The model under review builds one solid part; all positions refer to its coordinate system, in mm. Face numbers are marked on the shaded views. A direction names the side the tool comes from. Coordinates: 2 decimals unless noted, no trailing zeros. Write each loop counter-clockwise with the first axis right and the second up, starting at its lowest first coordinate (ties: lowest second). Pieces come first, ordered by that corner, then holes. Notation, with made-up numbers: (-36.75, 6) - (19.25, 6) arc R27 cw to (19.25, 33) - close; hole circle Ø3 at (-18.5, -5). An arc over 180 degrees is marked (long way). Return JSON: item names as keys, results as strings. Group by question number.
(1) For pin 1 Ø8 at (x, y) = (9, 45) entering from +Z; pin 2 Ø1 at (x, y) = (6.5, 98.5) entering from +Z; pin 3 Ø4 at (x, y) = (3, 37) entering from +Z; pin 4 Ø2.5 at (y, z) = (49.4, 132.79) entering from -X, all flat-tipped, find the tip position at first contact; note any pin that passes through.
(2) We need section C-C on y = 40.5. State the section outline as (x, z) points, then the cut area to 3 significant figures.
(3) Tool access review of the marked faces 4 and 5: name each direction out of +Z, -Z, +X, -X, +Y, -Y from which nothing blocks a thin tool from reaching the whole face with its end or side.
(4) Draft analysis for pull direction Z (two halves, no side actions). For the marked faces 1, 2 and 3, state which applies: released by +Z, released by -Z, zero draft, split by the parting line, or undercut.
(5) We need section A-A on x = 5.25. State the section outline as (y, z) points, then the cut area to 3 significant figures.
(6) To check wall thickness, follow L1, parallel to X at y = 108.5, z = 24; L2, parallel to Z at x = 12.5, y = 75; L3, parallel to Y at x = 1.75, z = 141.5. State the ranges of each line that lie inside material, in increasing order. Write a range as from..to.
(7) We need section B-B on z = 72. State the section outline as (x, y) points.
Autodesk Inventor part; units mm, degrees
ref_plane "YZ Plane" through (0, 0, 0) normal (1, 0, 0) x (0, 1, 0)
ref_plane "XZ Plane" through (0, 0, 0) normal (0, 1, 0) x (-1, 0, 0)
ref_plane "XY Plane" through (0, 0, 0) normal (0, 0, 1) x (1, 0, 0)
sketch "スケッチ1" plane through (0, 0, 0) normal (1, 0, 0) x (0, 1, 0)
  circle A0 centre (71.3451, 9.7822) radius 120
  line L0 (71.3451, 9.7822) -> (-260.1174, 9.7822) construction
  line L1 (138.8451, -107.1313) -> (-63.6549, 9.7822)
  circle A1 centre (71.3451, 9.7822) radius 5
  line L2 (71.3451, 9.7822) -> (138.8451, 126.6956) construction
  line L3 (71.3451, 9.7822) -> (138.8451, -107.1313) construction
  line L4 (71.3451, 9.7822) -> (-63.6549, 9.7822)
  line L5 (88.381, 47.2892) -> (83.381, 38.629) construction
  line L6 (83.381, 38.629) -> (86.8451, 36.629) construction
  line L7 (86.8451, 36.629) -> (91.8451, 45.2892) construction
  line L8 (91.8451, 45.2892) -> (88.381, 47.2892)
  line L9 (91.8451, 45.2892) -> (86.8451, 36.629) construction
  line L10 (86.8451, 36.629) -> (90.3092, 34.629) construction
  line L11 (90.3092, 34.629) -> (95.3092, 43.2892) construction
  line L12 (95.3092, 43.2892) -> (91.8451, 45.2892)
  line L13 (85.881, 42.9591) -> (92.8092, 38.9591) construction
  circle A2 centre (71.3451, 9.7822) radius 2.65 construction
  line L14 (88.1645, 47.4142) -> (81.6645, 36.1559) construction
  line L15 (81.6645, 36.1559) -> (77.3344, 38.6559) construction
  line L16 (77.3344, 38.6559) -> (83.8344, 49.9142) construction
  line L17 (83.8344, 49.9142) -> (88.1645, 47.4142)
  line L18 (95.5257, 43.1642) -> (89.0257, 31.9059) construction
  line L19 (89.0257, 31.9059) -> (93.3559, 29.4059) construction
  line L20 (93.3559, 29.4059) -> (99.8559, 40.6642) construction
  line L21 (99.8559, 40.6642) -> (95.5257, 43.1642)
  circle A3 centre (71.3451, 9.7822) radius 28.3207 construction
  line L22 (30.3451, 19.0322) -> (30.3451, 14.0322)
  line L23 (30.3451, 14.0322) -> (43.3451, 14.0322) construction
  line L24 (43.3451, 19.0322) -> (30.3451, 19.0322) construction
  line L25 (43.3451, 14.0322) -> (43.3451, 19.0322)
  line L26 (30.3451, 5.5322) -> (43.3451, 5.5322) construction
  line L27 (30.3451, 0.5322) -> (30.3451, 5.5322)
  line L28 (43.3451, 0.5322) -> (30.3451, 0.5322) construction
  line L29 (43.3451, 5.5322) -> (43.3451, 0.5322)
  line L30 (83.8344, -30.3499) -> (88.1645, -27.8499)
  line L31 (88.1645, -27.8499) -> (81.6645, -16.5915) construction
  line L32 (77.3344, -19.0915) -> (83.8344, -30.3499) construction
  line L33 (81.6645, -16.5915) -> (77.3344, -19.0915) construction
  line L34 (95.5257, -23.5999) -> (89.0257, -12.3415) construction
  line L35 (99.8559, -21.0999) -> (95.5257, -23.5999)
  line L36 (93.3559, -9.8415) -> (99.8559, -21.0999) construction
  line L37 (89.0257, -12.3415) -> (93.3559, -9.8415) construction
  line L38 (77.3344, 38.6559) -> (76.7181, 37.5885)
  line L39 (93.3559, 29.4059) -> (92.7396, 28.3385) construction
  line L40 (43.3451, 19.0322) -> (44.5776, 19.0322)
  line L41 (43.3451, 0.5322) -> (44.5776, 0.5322)
  line L42 (77.3344, -19.0915) -> (73.5386, -12.517) construction
  line L43 (93.3559, -9.8415) -> (92.7396, -8.7742) construction
  line L44 (84.956, 41.3569) -> (74.956, 24.0364) construction
  line L45 (74.956, 24.0364) -> (69.7599, 27.0364) construction
  line L46 (69.7599, 27.0364) -> (79.7599, 44.3569) construction
  line L47 (79.7599, 44.3569) -> (84.956, 41.3569)
  circle A4 centre (74.8579, 29.8666) radius 1.5
  circle A5 centre (79.8579, 38.5268) radius 1.5
  circle A6 centre (86.9823, 22.8666) radius 1.5
  circle A7 centre (91.9823, 31.5268) radius 1.5
  circle A8 centre (42.1951, 16.7822) radius 1.5
  circle A9 centre (52.1951, 16.7822) radius 1.5
  circle A10 centre (52.1951, 2.7822) radius 1.5
  circle A11 centre (42.1951, 2.7822) radius 1.5
  circle A12 centre (79.8579, -18.9625) radius 1.5
  circle A13 centre (74.8579, -10.3022) radius 1.5
  circle A14 centre (86.9823, -3.3022) radius 1.5
  circle A15 centre (91.9823, -11.9625) radius 1.5
  line L48 (72.3579, 25.5364) -> (84.956, 41.3569) construction
  circle A16 centre (71.3451, 9.7822) radius 34.3835
  line L49 (63.3451, 56.7822) -> (-116.6549, 56.7822) construction
  line L50 (-116.6549, 56.7822) -> (-116.6549, 41.7822)
  line L51 (-116.6549, 41.7822) -> (63.3451, 41.7822) construction
  line L52 (63.3451, 41.7822) -> (63.3451, 56.7822) construction
  circle A17 centre (53.3451, 49.2822) radius 1.5 construction
  circle A18 centre (43.3451, 49.2822) radius 1.5 construction
  line L53 (36.9617, 56.7822) -> (36.9617, 9.7822) construction
  line L54 (63.3451, 56.7822) -> (90.6652, 38.2244) construction
  line L55 (36.9617, -37.2178) -> (36.9617, 9.7822) construction
  line L56 (63.3451, -37.2178) -> (90.6652, -18.66) construction
  line L57 (63.3451, -37.2178) -> (-116.6549, -37.2178) construction
  line L58 (-116.6549, -22.2178) -> (63.3451, -22.2178) construction
  circle A19 centre (43.3451, -29.7178) radius 1.5 construction
  circle A20 centre (53.3451, -29.7178) radius 1.5 construction
  line L59 (71.3451, 9.7822) -> (54.1534, 39.5591)
  line L60 (62.8136, 44.5591) -> (45.4931, 34.5591)
  line L61 (45.4931, 34.5591) -> (50.4931, 25.8989)
  line L62 (50.4931, 25.8989) -> (67.8136, 35.8989)
  line L63 (67.8136, 35.8989) -> (62.8136, 44.5591)
  circle A21 centre (60.9835, 37.729) radius 1.5
  circle A22 centre (52.3233, 32.729) radius 1.5
  circle A23 centre (52.3233, -13.1647) radius 1.5
  circle A24 centre (60.9835, -18.1647) radius 1.5
  circle A25 centre (100.7286, 4.7822) radius 1.5
  circle A26 centre (100.7286, 14.7822) radius 1.5
  circle A27 centre (71.3451, 9.7822) radius 193.5
  line L64 (-121.5196, 25.4487) -> (154.2099, 184.6412)
  line L65 (71.3451, 9.7822) -> (11.3451, 113.7052)
  line L66 (71.3451, 9.7822) -> (71.3451, 203.2822)
  line L67 (124.6464, 17.4617) -> (23.1464, 193.2648)
  line L68 (23.1464, 193.2648) -> (10.156, 185.7648)
  line L69 (10.156, 185.7648) -> (111.656, 9.9617)
  line L70 (111.656, 9.9617) -> (124.6464, 17.4617)
  circle A28 centre (49.4012, 132.7902) radius 1.5
  circle A29 centre (20.4012, 183.0196) radius 1.5
  circle A30 centre (62.2784, 25.4862) radius 1.5
  circle A31 centre (71.3451, 9.7822) radius 12.5
  circle A32 centre (62.2784, -5.9219) radius 1.5
  circle A33 centre (89.4786, 9.7822) radius 1.5
  circle A34 centre (113.1512, 22.3719) radius 1.5
  circle A35 centre (103.1512, 39.6924) radius 1.5
  circle A36 centre (71.3451, 9.7822) radius 24.3835
  line L71 (124.6464, 17.4617) -> (93.4246, -0.5642)
  line L72 (104.6464, 52.1027) -> (73.4246, 34.0768)
  line L73 (18.0439, 2.1027) -> (49.2656, 20.1286)
  circle A37 centre (29.539, -2.8076) radius 1.5
  circle A38 centre (39.539, -20.1281) radius 1.5
  line L74 (38.0439, -32.5383) -> (-63.4561, 143.2648)
  line L75 (51.0342, -25.0383) -> (38.0439, -32.5383)
  line L76 (38.0439, -32.5383) -> (69.2656, -14.5125)
  point P0 (0, 0)
  point P1 (90.9669, 45.7962)
  point P2 (92.3451, 45.0005)
  point P3 (91.656, 44.6027)
  dimension "d4" = 3
  dimension "d5" = 3
  dimension "d6" = 10
  dimension "d7" = 10
  dimension "d8" = 7.5
  dimension "d9" = 7.5
  dimension "d10" = 60
  dimension "d11" = 10
  dimension "d12" = 10
  dimension "d13" = 10
  dimension "d14" = 3
  dimension "d15" = 5
  dimension "d16" = 5
  dimension "d17" = 360
  dimension "d18" = 387
  dimension "d19" = 110
  dimension "d20" = 60
  dimension "d21" = 15
  dimension "d22" = 73
  dimension "d23" = 3
  dimension "d24" = 3
  dimension "d25" = 7.5
  dimension "d26" = 7.5
  dimension "d27" = 7.5
  dimension "d28" = 7.5
  dimension "d29" = 3
  dimension "d30" = 25
  dimension "d31" = 6.25
  dimension "d32" = 360
  dimension "d33" = 20
  dimension "d34" = 3
  dimension "d35" = 3
  dimension "d36" = 10
  dimension "d37" = 7.5
  dimension "d38" = 7.5
  dimension "d39" = 20
  dimension "d40" = 35
  dimension "d41" = 10
extrude "押し出し1" add sketch "スケッチ1" along normal blind 15 contours L67 L66 L69 L64 A0 | A0 L64 L67 | L67 L72 L12 L8 L69 L66 | L64 L69 A0 | A0 L69 L68 L67 L64 | L67 L70 L69 L72 | L8 L12 L72 L69 | A28 | A29 | A34 | A35
shell "シェル1" thickness 1 removed faces 2 at (5, 18.8163, 190.7648) at (5, 115.9861, 12.4617)
hole "穴1" at (0, 138.8451, 126.6956) at (0, -63.6549, 9.7822) at (0, 138.8451, -107.1313) at (0, 20.4012, 183.0196) at (0, 49.4012, 132.7902) at (0, 103.1512, 39.6924) at (0, 113.1512, 22.3719) direction (1, 0, 0) diameter 3.4 end through all
equation "\"d9\" = d8"
properties part number "hand-grab-v3-ASP_1" material "アルミニウム 6061"
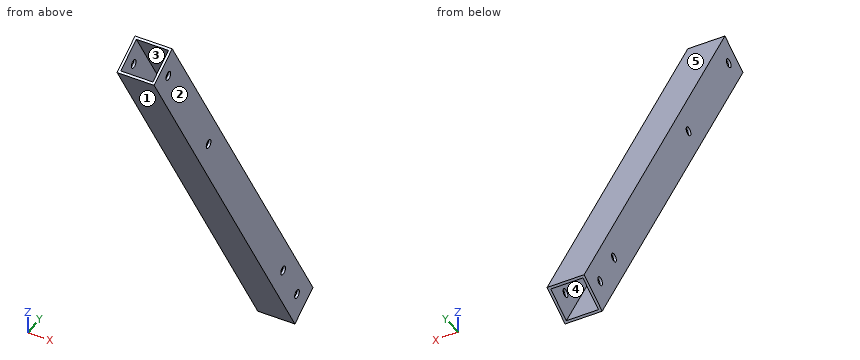
Ans:
{
 "1": {"pin 1": "z = 162.34", "pin 2": "z = 63.61", "pin 3": "z = 172.73", "pin 4": "through"},
 "2": {"outline": "(0, 133.21) - (15, 133.21) - (15, 163.21) - (0, 163.21) - close; hole (1, 135.21) - (14, 135.21) - (14, 161.21) - (1, 161.21) - close", "area": "112 mm²"},
 "3": {"face 4": "none", "face 5": "+Z, +X, -X, +Y"},
 "4": {"face 1": "released by -Z", "face 2": "zero draft", "face 3": "undercut"},
 "5": {"outline": "(10.16, 185.76) - (111.66, 9.96) - (112.52, 10.46) - (11.02, 186.26) - close; (22.28, 192.76) - (123.78, 16.96) - (124.65, 17.46) - (23.15, 193.26) - close", "area": "406 mm²"},
 "6": {"L1": "0..1, 14..15", "L2": "73.45..75.45, 101.45..103.45", "L3": "35.71..36.87, 51.88..53.03"},
 "7": {"outline": "(0, 75.84) - (15, 75.84) - (15, 93.16) - (0, 93.16) - close; hole (1, 76.99) - (14, 76.99) - (14, 92) - (1, 92) - close"}
}
